Geometry check sheet. Reference: the model listing, model coordinates, mm. A direction names the side the tool comes from. Round coordinates to 2 decimals unless told otherwise and drop trailing zeros. Order: outer loops, then holes, each group sorted by start corner. A loop starts at its lowest first (then second) coordinate and runs counter-clockwise, first axis right, second up. Notation, with made-up numbers: (-7, 18.25) - (28, 18.25) arc R9 ccw to (28, 22.25) - close; hole circle Ø8 at (37.25, 15.5). An arc over 180 degrees is marked (long way). Write each question's results on one line, items separated by ' | '.
```python
from build123d import *

# Parameters (mm, degrees)
SKETCH1_R                           = 9.5
BOSS_EXTRUDE1_DEPTH                 = 20
SKETCH2_OUTSIDE_W                   = 27.7
SKETCH2_OUTSIDE_H                   = 27.7
SKETCH2_OUTSIDE_R                   = 8
CUT_EXTRUDE1_DEPTH                  = 18
SKETCH3_OUTSIDE_W                   = 27.7
SKETCH3_OUTSIDE_H                   = 27.7
SKETCH3_OUTSIDE_R                   = 6
CUT_EXTRUDE2_DEPTH                  = 13
SKETCH4_OUTSIDE_W                   = 27.7
SKETCH4_OUTSIDE_H                   = 27.7
SKETCH4_OUTSIDE_R                   = 5.5
CUT_EXTRUDE3_DEPTH                  = 5.5
SKETCH5_W                           = 1
SKETCH5_H                           = 0.5
CHAMFER1_SIZE                       = 0.3
CHAMFER2_SIZE                       = 1.3
SKETCH7_R                           = 4.05
CUT_EXTRUDE4_DEPTH                  = 25.093567606
SKETCH8_R                           = 4.5
CUT_EXTRUDE5_DEPTH                  = 4.5
SKETCH9_R                           = 4.45
CUT_EXTRUDE9_DEPTH                  = 0.2
SKETCH10_R                          = 7
CUT_EXTRUDE11_DEPTH                 = 6
CUT_EXTRUDE12_START                 = -5.6
SKETCH11_R                          = 5.5
CUT_EXTRUDE12_DEPTH                 = 5.6
SKETCH12_R                          = 5.25
CUT_EXTRUDE13_DEPTH                 = 1.9
CHAMFER3_SIZE                       = 1.2
F_1_2_1_2_DIAMETER_HOLE1_AT_2_COUNT = 2
F_1_2_1_2_DIAMETER_HOLE1_AT_2_PITCH = 14


with BuildPart() as part:
    # Sketch1 → Boss-Extrude1 (new body)
    with BuildSketch(Plane.XY):
        Circle(SKETCH1_R)
    extrude(amount=-BOSS_EXTRUDE1_DEPTH)

    # Sketch2 outside → Cut-Extrude1 (cut)
    with BuildSketch(Plane(origin=(0, 0, -20), x_dir=(-1, 0, 0), z_dir=(0, 0, -1))):
        Rectangle(SKETCH2_OUTSIDE_W, SKETCH2_OUTSIDE_H)
        Circle(SKETCH2_OUTSIDE_R, mode=Mode.SUBTRACT)
    extrude(amount=-CUT_EXTRUDE1_DEPTH, mode=Mode.SUBTRACT)

    # Sketch3 outside → Cut-Extrude2 (cut)
    with BuildSketch(Plane(origin=(0, 0, -20), x_dir=(-1, 0, 0), z_dir=(0, 0, -1))):
        Rectangle(SKETCH3_OUTSIDE_W, SKETCH3_OUTSIDE_H)
        Circle(SKETCH3_OUTSIDE_R, mode=Mode.SUBTRACT)
    extrude(amount=-CUT_EXTRUDE2_DEPTH, mode=Mode.SUBTRACT)

    # Sketch4 outside → Cut-Extrude3 (cut)
    with BuildSketch(Plane(origin=(0, 0, -20), x_dir=(-1, 0, 0), z_dir=(0, 0, -1))):
        Rectangle(SKETCH4_OUTSIDE_W, SKETCH4_OUTSIDE_H)
        Circle(SKETCH4_OUTSIDE_R, mode=Mode.SUBTRACT)
    extrude(amount=-CUT_EXTRUDE3_DEPTH, mode=Mode.SUBTRACT)

    # Sketch5 → Cut-Revolve1 (revolve, cut)
    with BuildSketch(Plane(origin=(0, 0, 0), x_dir=(0, 0, -1), z_dir=(1, 0, 0)), mode=Mode.PRIVATE) as cut_revolve1_sk:
        with Locations((15, 5.25)):
            Rectangle(SKETCH5_W, SKETCH5_H)
    revolve(cut_revolve1_sk.sketch.rotate(Axis((0, 0, 0), (0, 0, -1)), 90), axis=Axis((0, 0, 0), (0, 0, -1)), mode=Mode.SUBTRACT)

    # Chamfer1
    chamfer1_edges = [part.edges().sort_by_distance(p)[0] for p in [
        (5.5, 0, -20),
    ]]
    chamfer(chamfer1_edges, length=CHAMFER1_SIZE)

    # Chamfer2
    chamfer2_edges = [part.edges().sort_by_distance(p)[0] for p in [
        (-9.5, 0, 0),
    ]]
    chamfer(chamfer2_edges, length=CHAMFER2_SIZE)

    # Sketch6 → Cut-Revolve2 (revolve, cut)
    with BuildSketch(Plane(origin=(0, 0, 0), x_dir=(0, 0, -1), z_dir=(1, 0, 0)), mode=Mode.PRIVATE) as cut_revolve2_sk:
        with BuildLine():
            Line((7.2, -7.033012702), (6.776794919, -6.3))
            ThreePointArc((6.776794919, -6.3), (6.776794919, -6.1), (6.95, -6))
            Line((6.95, -6), (7.2, -6))
            Line((7.2, -6), (7.2, -7.033012702))
        make_face()
    revolve(cut_revolve2_sk.sketch.rotate(Axis((0, 0, 0), (0, 0, -1)), 270), axis=Axis((0, 0, 0), (0, 0, -1)), mode=Mode.SUBTRACT)

    # Sketch7 → Cut-Extrude4 (cut, through all)
    with BuildSketch(Plane.XY):
        Circle(SKETCH7_R)
    extrude(amount=-CUT_EXTRUDE4_DEPTH, mode=Mode.SUBTRACT)

    # Sketch8 → Cut-Extrude5 (cut)
    with BuildSketch(Plane(origin=(0, 0, -20), x_dir=(-1, 0, 0), z_dir=(0, 0, -1))):
        Circle(SKETCH8_R)
    extrude(amount=-CUT_EXTRUDE5_DEPTH, mode=Mode.SUBTRACT)

    # Sketch9 → Cut-Extrude9 (cut)
    with BuildSketch(Plane(origin=(0, 0, -15.5), x_dir=(-1, 0, 0), z_dir=(0, 0, -1))):
        Circle(SKETCH9_R)
    extrude(amount=-CUT_EXTRUDE9_DEPTH, mode=Mode.SUBTRACT)

    # Sketch10 → Cut-Extrude11 (cut)
    with BuildSketch(Plane.XY):
        Circle(SKETCH10_R)
    extrude(amount=-CUT_EXTRUDE11_DEPTH, mode=Mode.SUBTRACT)

    # Sketch11 → Cut-Extrude12 (cut)
    with BuildSketch(Plane.XY.offset(-6).offset(CUT_EXTRUDE12_START)):
        Circle(SKETCH11_R)
    extrude(amount=CUT_EXTRUDE12_DEPTH, mode=Mode.SUBTRACT)

    # Sketch12 → Cut-Extrude13 (cut)
    with BuildSketch(Plane.XY.offset(-11.6)):
        Circle(SKETCH12_R)
    extrude(amount=-CUT_EXTRUDE13_DEPTH, mode=Mode.SUBTRACT)

    # Chamfer3
    chamfer3_edges = [part.edges().sort_by_distance(p)[0] for p in [
        (-4.05, 0, -13.5),
    ]]
    chamfer(chamfer3_edges, length=CHAMFER3_SIZE - 0.0001)  # a hair under: the kernel refuses the full size

    # Sketch15 → Ø1.2 (1.2) Diameter Hole1 (revolve, cut)
    with BuildSketch(Plane(origin=(0, -7, -7), x_dir=(0, 1, 0), z_dir=(1, 0, 0))):
        Polygon((0, 0), (0, 1.360516371), (0.6, 1), (0.6, 0), align=None)
    f_1_2_1_2_diameter_hole1 = revolve(axis=Axis((0, -7, -13.35), (0, 0, 1)), mode=Mode.SUBTRACT)

    # Ø1.2 (1.2) Diameter Hole1 at 2: Ø1.2 (1.2) Diameter Hole1 ×2
    with Locations(*[(0, i * F_1_2_1_2_DIAMETER_HOLE1_AT_2_PITCH, 0) for i in range(1, F_1_2_1_2_DIAMETER_HOLE1_AT_2_COUNT)]):
        add(f_1_2_1_2_diameter_hole1, mode=Mode.SUBTRACT)


solid = part.part
```
(1) Access from +Z, -Z, +X, -X, +Y, -Y to the whole of each face (thin tool, end or side, straight path). Record for faces 1 (the face through (-4, 4, -6)), 2 (the face through (-1.6, 4.9, -15.5)), 3 (the face through (4.3, -7, -2)).
Answers follow:
face 1: +Z | face 2: none | face 3: -Z
(2) Section check C-C (z = -15). Record the cut outline in (x, y).
Answers follow:
outline: circle Ø10 at (0, 0); hole circle Ø8.1 at (0, 0)
(3) Draft check along Y on faces 4 (the face through (1.73, -7.81, -4.54)), 5 (the face through (-0.878, -3.954, -14.996)), 6 (the face through (-3.1, 3.5, -20)). Enter one of: released by +Y, released by -Y, zero draft, split by the parting line, or undercut.
Answers follow:
face 4: split by the parting line | face 5: undercut | face 6: zero draft
(4) Section check A-A (z = -3.75). Record the cut outline in (x, y).
Answers follow:
outline: circle Ø16 at (0, 0); hole circle Ø14 at (0, 0)
(5) Depth check by flat-ended pin: pin 1 Ø8.5 at (x, y) = (-1.5, 0.5) entering from +Z; pin 2 Ø9.5 at (x, y) = (0, 0) entering from +Z; pin 3 Ø4 at (y, z) = (2.5, -7) entering from +X. Enter the tip coordinate at first touch or a pass-through.
Answers follow:
pin 1: z = -6 | pin 2: z = -14 | pin 3: x = 7.98
(6) Material ranges on line 1 (Y direction, x = 0, z = -6.65); line 2 (Y direction, x = 0, z = -12.75); line 3 (Y direction, x = 0, z = -18.85), recorded low to high.
Answers follow:
line 1: -8 to -7.6, -6.4 to -5.5, 5.5 to 6.4, 7.6 to 8 | line 2: -6 to -5.25, 5.25 to 6 | line 3: -5.5 to -4.5, 4.5 to 5.5
